from build123d import *

# Parameters (mm, degrees)
SKETCH1_R           = 4.7879
SKETCH1_R_2         = 3.1877
BOSS_EXTRUDE1_DEPTH = 6.4135
FILLET1_R           = 12.7


with BuildPart() as part:
    # Sketch1 → Boss-Extrude1 (new body, symmetric)
    with BuildSketch(Plane.XY):
        Polygon((0, 0), (22.352, 0), (88.9, 24.22149115), (88.9, 50.8), (0, 50.8), align=None)
        with Locations((16.51, 12.7)):
            Circle(SKETCH1_R, mode=Mode.SUBTRACT)
        with Locations((16.51, 38.1)):
            Circle(SKETCH1_R, mode=Mode.SUBTRACT)
        with Locations((67.31, 38.1)):
            Circle(SKETCH1_R, mode=Mode.SUBTRACT)
        with Locations((41.91, 25.4)):
            Circle(SKETCH1_R_2, mode=Mode.SUBTRACT)
    extrude(amount=BOSS_EXTRUDE1_DEPTH, both=True)

    # Fillet1
    fillet1_edges = [part.edges().sort_by_distance(p)[0] for p in [
        (88.9, 24.22149115, 0),
        (22.352, 0, 0),
    ]]
    fillet(fillet1_edges, radius=FILLET1_R)


solid = part.part
Verification items for the finished model (mm, model axes). Give positions to 0.01 mm unless a question says otherwise; leave off trailing zeros. Order: outer loops, then holes, each group sorted by start corner. A loop starts at its lowest first (then second) coordinate and runs counter-clockwise, first axis right, second up. Notation, with made-up numbers: (45.25, 43.25) -> (75.25, 43.25) arc R14 cw to (75.25, 52.25) -> close; hole circle Ø11 at (38, 80.25). An arc over 180 degrees is marked (long way). Answer as CSV lines item,"result".
Q1. Sectioned sample at A-A on x = 16.51. Record the cut outline in (y, z), plus the area to 3 significant figures.
Solutions:
outline,"(0, -6.41) -> (7.91, -6.41) -> (7.91, 6.41) -> (0, 6.41) -> close; (17.49, -6.41) -> (33.31, -6.41) -> (33.31, 6.41) -> (17.49, 6.41) -> close; (42.89, -6.41) -> (50.8, -6.41) -> (50.8, 6.41) -> (42.89, 6.41) -> close"
area,"406 mm²"
Q2. Sectioned sample at B-B on z = -4.25. Record the cut outline in (x, y), plus the area to 3 significant figures.
Solutions:
outline,"(0, 0) -> (20.11, 0) arc R12.7 ccw to (24.46, 0.77) -> (80.54, 21.18) arc R12.7 ccw to (88.9, 33.11) -> (88.9, 50.8) -> (0, 50.8) -> close; hole circle Ø9.58 at (16.51, 12.7); hole circle Ø9.58 at (16.51, 38.1); hole circle Ø6.38 at (41.91, 25.4); hole circle Ø9.58 at (67.31, 38.1)"
area,"3,450 mm²"
Q3. Depth check by flat-ended pin: pin 1 (4 mm diameter, centred on x = 51.5, z = 0, fed in from -Y); pin 2 (7.5 mm diameter, centred on x = 16.51, y = 38.1, fed in from -Z); pin 3 (3 mm diameter, centred on x = 37, z = -4.5, fed in from -Y). Enter the tip coordinate at first touch or a pass-through.
Solutions:
pin 1,"stops at y = 9.88"
pin 2,"passes through"
pin 3,"stops at y = 4.79"
Q4. Release check for a two-part mould opening along X. For faces 1 (the flat face through (52.11, 10.83, 0.09)), 2 (the flat face through (45, 50.8, 0)), 3 (the cylindrical face through (63.781, 41.336, -0.09)) record: +X half, -X half, draft (parallel to the pull), parting line (faces both ways), or undercut.
Solutions:
face 1,"+X half"
face 2,"draft"
face 3,"undercut"
Q5. Sectioned sample at D-D on x = 41.91. Record the cut outline in (y, z), plus the area to 3 significant figures.
Solutions:
outline,"(7.12, -6.41) -> (22.21, -6.41) -> (22.21, 6.41) -> (7.12, 6.41) -> close; (28.59, -6.41) -> (50.8, -6.41) -> (50.8, 6.41) -> (28.59, 6.41) -> close"
area,"479 mm²"
Q6. Sectioned sample at C-C on y = 12.7. Record the cut outline in (x, z), plus the area to 3 significant figures.
Solutions:
outline,"(0, -6.41) -> (11.72, -6.41) -> (11.72, 6.41) -> (0, 6.41) -> close; (21.3, -6.41) -> (57.24, -6.41) -> (57.24, 6.41) -> (21.3, 6.41) -> close"
area,"611 mm²"
Q7. Scan lines: probe 1 along Y at (x, z) = (16.51, 0); probe 2 along X at (y, z) = (34, 0.5); probe 3 along X at (y, z) = (33, 2.75). Record each from-to range of solid material in increasing order.
Solutions:
probe 1,"y = 0 to 7.91, 17.49 to 33.31, 42.89 to 50.8"
probe 2,"x = 0 to 14.04, 18.98 to 64.84, 69.78 to 88.9"
probe 3,"x = 0 to 88.9"
